The model under review builds one solid part; all positions refer to its coordinate system, in mm. Face numbers are marked on the shaded views. A direction names the side the tool comes from. Coordinates: 2 decimals unless noted, no trailing zeros. Order: outer loops, then holes, each group sorted by start corner. A loop starts at its lowest first (then second) coordinate and runs counter-clockwise, first axis right, second up. Notation, with made-up numbers: (59, 37.5) -> (88, 37.5) arc R27 cw to (88, 59.5) -> close; hole circle Ø6 at (1.25, -11.5). An arc over 180 degrees is marked (long way). Use CSV: the item, a comma, the result in double quotes. Start each with the question number.
```python
from build123d import *

# Parameters (mm, degrees)
F1_DEPTH = 50
F2_R     = 7.14375
F3_DEPTH = 50.801


with BuildPart() as f1:
    # F0 (on Right) → F1 (new body, symmetric)
    with BuildSketch(Plane.YZ):
        Polygon((0, -42.8625), (0, 0), (44.45, 0), (44.45, -42.8625), (47.625, -42.8625), (47.625, 3.175), (-3.175, 3.175), (-3.175, -42.8625), align=None)
    extrude(amount=F1_DEPTH, both=True)

    # F2 (on face) → F3 (cut, through all)
    with BuildSketch(Plane(origin=(0, 47.625, 0), x_dir=(-1, 0, 0), z_dir=(0, 1, 0))):
        with Locations((-29.0336, -19.84375)):
            Circle(F2_R)
        with Locations((29.2414, -19.84375)):
            Circle(F2_R)
    extrude(amount=-F3_DEPTH, mode=Mode.SUBTRACT)


solid = f1.part
```
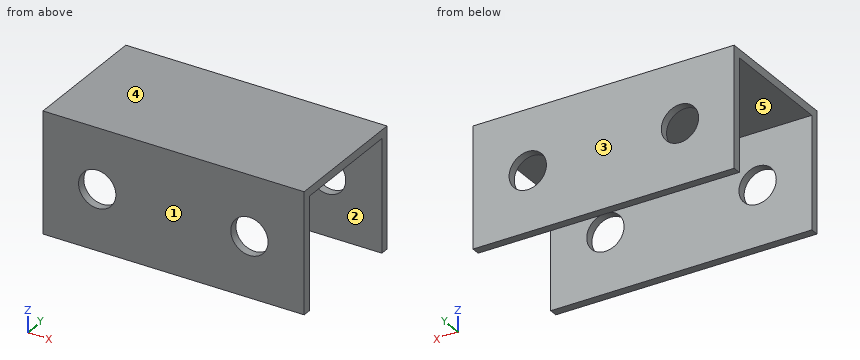
Q1. Draft analysis for pull direction Y (two halves, no side actions). For the marked faces 1, 2 and 3, state which applies: +Y half, -Y half, draft (parallel to the pull), parting line (faces both ways), or undercut.
Q2. Add section A-A, the plane z = -6.5. State the section outline as (x, y) points (3 decimals), then the cut area to 3 significant figures.
Q3. Clearance check with flat-ended pins moving along their axes: pin 1 Ø13 at (x, z) = (-29.24, -19.84) entering from -Y; pin 2 Ø6 at (x, y) = (-33.5, 27.5) entering from -Z. State where each tip first meets the part, or that it passes through.
Q4. To check wall thickness, follow probe 1 along Y at (x, z) = (-40.5, -24) (3 decimals); probe 2 along Z at (x, y) = (-20.5, 41) (3 decimals). State the ranges of each line that lie inside material, in increasing order.
Q5. Add section C-C, the plane z = -14. State the section outline as (x, y) points (3 decimals).
Q6. For the marked faces 4 and 5, list the 3-axis set-ups (+Z, -Z, +X, -X, +Y, -Y) from which the entire face can be reached by the end or side of a thin tool; tool diameter is ignored.
Q7. Add section B-B, the plane x = -31. State how many separate pieces and enclosed holes the cut face has, then the cut area to 3 significant figures.
Answer block:
1,face 1,"-Y half"
1,face 2,"undercut"
1,face 3,"+Y half"
2,outline,"(-50, -3.175) -> (50, -3.175) -> (50, 0) -> (-50, 0) -> close; (-50, 44.45) -> (50, 44.45) -> (50, 47.625) -> (-50, 47.625) -> close"
2,area,"635 mm²"
3,pin 1,"passes through"
3,pin 2,"stops at z = 0"
4,probe 1,"y = -3.175 to 0, 44.45 to 47.625"
4,probe 2,"z = 0 to 3.175"
5,outline,"(-50, -3.175) -> (-33.35, -3.175) -> (-33.35, 0) -> (-50, 0) -> close; (-50, 44.45) -> (-33.35, 44.45) -> (-33.35, 47.625) -> (-50, 47.625) -> close; (-25.132, -3.175) -> (24.925, -3.175) -> (24.925, 0) -> (-25.132, 0) -> close; (-25.132, 44.45) -> (24.925, 44.45) -> (24.925, 47.625) -> (-25.132, 47.625) -> close; (33.143, -3.175) -> (50, -3.175) -> (50, 0) -> (33.143, 0) -> close; (33.143, 44.45) -> (50, 44.45) -> (50, 47.625) -> (33.143, 47.625) -> close"
6,face 4,"+Z, +X, -X, +Y, -Y"
6,face 5,"-Z, +X, -X"
7,separate pieces,"3"
7,enclosed holes,"0"
7,area,"346 mm²"
